Autodesk Inventor part; units mm, degrees
ref_plane "YZ Plane" through (0, 0, 0) normal (1, 0, 0) x (0, 1, 0)
ref_plane "XZ Plane" through (0, 0, 0) normal (0, 1, 0) x (-1, 0, 0)
ref_plane "XY Plane" through (0, 0, 0) normal (0, 0, 1) x (1, 0, 0)
sketch "Boceto1" plane through (0, 0, 0) normal (0, 0, 1) x (1, 0, 0)
  line L0 (0, 0) -> (50, 0)
  line L1 (50, 0) -> (50, 50)
  line L2 (50, 50) -> (0, 50)
  line L3 (0, 50) -> (0, 0)
  line L4 (50, 0) -> (0, 0)
  line L5 (0, 0) -> (0, 10)
  line L6 (0, 10) -> (50, 10)
  line L7 (50, 10) -> (50, 0)
  dimension "d0" = 50
  dimension "d1" = 50
  dimension "d2" = 10
extrude "Extrusión1" add sketch "Boceto1" along normal blind 10
sketch "Boceto2" plane through (0, 0, 10) normal (0, 0, 1) x (1, 0, 0)
  line L0 (0, 0) -> (50, 0)
  line L1 (0, 50) -> (0, 0)
  line L2 (50, 0) -> (0, 0)
  line L3 (0, 0) -> (0, 10)
  line L4 (0, 10) -> (50, 10)
  line L5 (50, 10) -> (50, 0)
  dimension "d5" = 10
extrude "Extrusión2" add sketch "Boceto2" along normal blind 30
sketch "Boceto3" plane through (0, 0, 10) normal (0, 0, 1) x (1, 0, 0)
  circle A0 centre (25, 25) radius 3.4
  line L0 (0, 50) -> (0, 10)
  line L1 (0, 0) -> (50, 0)
  dimension "d8" = 6.8
  dimension "d9" = 25
  dimension "d10" = 25
extrude "Extrusión3" cut sketch "Boceto3" against normal blind 10
sketch "Boceto4" plane through (0, 10, 10) normal (0, 1, 0) x (1, 0, 0)
  circle A0 centre (25, -20) radius 5.1
  line L0 (50, 10) -> (0, 10)
  line L1 (0, 0) -> (0, -30)
  dimension "d13" = 10.2
  dimension "d14" = 30
  dimension "d15" = 25
extrude "Extrusión4" cut sketch "Boceto4" against normal blind 10
sketch "Boceto5" plane through (0, 0, 0) normal (-1, 0, 0) x (0, 0, 1)
  line L0 (0, 50) -> (10, 50)
  line L1 (10, 10) -> (40, 10)
  line L2 (10, 50) -> (40, 10)
  line L3 (40, 10) -> (10, 10)
  line L4 (10, 10) -> (10, 50)
  line L5 (10, 50) -> (10, 10)
  point P0 (0, 0)
extrude "Extrusión5" add sketch "Boceto5" against normal blind 5
sketch "Boceto6" plane through (50, 0, 0) normal (1, 0, 0) x (0, 0, -1)
  line L0 (-10, 50) -> (-40, 10)
  line L1 (-10, 10) -> (-40, 10)
  line L2 (-10, 50) -> (-40, 10)
  line L3 (-40, 10) -> (-10, 10)
  line L4 (-10, 50) -> (-10, 10)
  line L5 (-10, 10) -> (-10, 50)
  point P0 (0, 0)
sketch "Boceto7" plane through (50, 0, 0) normal (1, 0, 0) x (0, 0, -1)
  point P0 (0, 0)
sketch "Boceto8" plane through (0, 0, 10) normal (0, 0, 1) x (1, 0, 0)
  point P0 (0, 0)
extrude "Extrusión6" add sketch "Boceto6" against normal blind 5
sketch "Boceto9" plane through (0, 0, 0) normal (0, 0, -1) x (-1, 0, 0)
  line L0 (-5, 5) -> (-45, 5)
  line L1 (-45, 5) -> (-45, 45)
  line L2 (-45, 45) -> (-5, 45)
  line L3 (-5, 45) -> (-5, 5)
  line L4 (-50, 0) -> (-50, 50)
  line L5 (-50, 50) -> (0, 50)
  line L6 (0, 50) -> (0, 0)
  line L7 (0, 0) -> (-50, 0)
  line L8 (-50, 0) -> (-50, 50)
  line L9 (-50, 50) -> (0, 50)
  line L10 (0, 50) -> (0, 0)
extrude "Extrusión7" add sketch "Boceto9" along normal blind 20
sketch "Boceto10" plane through (50, 0, 40) normal (1, 0, 0) x (0, 0, -1)
  line L0 (0, 0) -> (0, 10)
  circle A0 centre (50, 25) radius 3.375
  line L1 (60, 0) -> (0, 0)
  line L2 (60, 50) -> (60, 0)
  point P0 (40, 0)
  dimension "d28" = 40
  dimension "d29" = 6.75
sketch "Boceto11" plane through (0, 0, 40) normal (0, -1, 0) x (1, 0, 0)
  circle A0 centre (25, -50) radius 3.375
  line L0 (0, -60) -> (0, 0)
  line L1 (50, -60) -> (0, -60)
  point P0 (0, -40)
  dimension "d32" = 6.75
sketch "Boceto12" plane through (0, 0, 40) normal (-1, 0, 0) x (0, 0, 1)
  circle A0 centre (-50, 25) radius 3.375
  line L0 (-60, 0) -> (-60, 50)
  line L1 (-30, 50) -> (-60, 50)
  point P0 (-40, 0)
  dimension "d35" = 6.75
sketch "Boceto13" plane through (0, 50, 10) normal (0, 1, 0) x (1, 0, 0)
  circle A0 centre (25, 20) radius 3.375
  line L0 (0, 30) -> (50, 30)
  line L1 (50, 30) -> (50, 0)
  point P0 (0, 10)
  dimension "d38" = 6.75
  dimension "d39" = 10
  dimension "d40" = 25
extrude "Extrusión8" cut sketch "Boceto13" against normal blind 5
extrude "Extrusión9" cut sketch "Boceto10" against normal blind 5
extrude "Extrusión10" cut sketch "Boceto11" against normal blind 5
extrude "Extrusión11" cut sketch "Boceto12" against normal blind 5
properties part number "UnionLlantaOmega" material "Plástico ABS"
Input: part model. Units: mm. Frame: model coordinates. A direction names the side the tool comes from. Give positions to 0.01 mm unless a question says otherwise; leave off trailing zeros. Write each loop counter-clockwise with the first axis right and the second up, starting at its lowest first coordinate (ties: lowest second). Pieces come first, ordered by that corner, then holes.
Q1. Set-up query: faces 1 (the face through (5, 21, 18)), 2 (the face through (25, 50, -5)), 3 (the face through (29, 5, -10)). Return all of +Z, -Z, +X, -X, +Y, -Y with unobstructed straight access to the full face (end or side cutting, diameter ignored); none if empty.
Q2. Material intervals for probe 1 along Z at (x, y) = (25, 4.5) (3 decimals); probe 2 along X at (y, z) = (21, 26), sorted ascending.
Q3. First-contact query: P1, Ø1, axis at x = 13, y = 38, coming from the +Z side; P2, Ø2, axis at x = 32.5, y = 23, coming from the -Z side; P3, Ø15, axis at x = 25.5, z = 20, coming from the +Y side; P4, Ø16, axis at y = 22.5, z = -10, coming from the -X side. Flat tips, straight axial feed; report the tip coordinate or a pass-through.
Q4. Section A-A, the plane x = 25. Output: boundary loops of the cut face in (y, z) (3 decimals), plus the area to 4 significant figures.
Q5. Section D-D, the plane y = 7.5. Output: boundary loops of the cut face in (x, z), plus the area to 3 significant figures.
Q6. Pull-direction query (X, two-part tool) for faces 4 (the face through (45, 29, -10)), 5 (the face through (0, 20, 4)), 6 (the face through (2, 30, 25)), 7 (the face through (20.95, 5.07, 33.1)); classes: pulls with the +X half, pulls with the -X half, needs draft (parallel to the pull), parting line crosses it, or undercut.
Q7. Section B-B, the plane y = 25. Output: boundary loops of the cut face in (x, z) (3 decimals), plus the area to 3 significant figures.
Q8. Section C-C, the plane z = -16. Output: boundary loops of the cut face in (x, y), plus the area to 3 significant figures.
Filled in:
1. face 1: +Z, +Y
1. face 2: +Z, -Z, +X, -X, +Y
1. face 3: -Z
2. probe 1: z = -20 to -13.375, -6.625 to 24.9, 35.1 to 40
2. probe 2: x = 0 to 5, 45 to 50
3. P1: stops at z = 10
3. P2: stops at z = 0
3. P3: stops at y = 10
3. P4: stops at x = 0
4. outline: (0, -20) - (5, -20) - (5, -13.375) - (0, -13.375) - close; (0, -6.625) - (5, -6.625) - (5, 0) - (21.6, 0) - (21.6, 10) - (10, 10) - (10, 24.9) - (0, 24.9) - close; (0, 35.1) - (10, 35.1) - (10, 40) - (0, 40) - close; (28.4, 0) - (45, 0) - (45, -6.625) - (50, -6.625) - (50, 10) - (28.4, 10) - close; (45, -20) - (50, -20) - (50, -13.375) - (45, -13.375) - close
4. area: 762.5 mm2
5. outline: (0, -20) - (5, -20) - (5, 0) - (45, 0) - (45, -20) - (50, -20) - (50, 40) - (0, 40) - close; hole circle Ø10.2 at (25, 30)
5. area: 2,120 mm2
6. face 4: undercut
6. face 5: pulls with the -X half
6. face 6: needs draft
6. face 7: undercut
7. outline: (0, -20) - (5, -20) - (5, -13.375) - (0, -13.375) - close; (0, -6.625) - (5, -6.625) - (5, 0) - (21.6, 0) - (21.6, 10) - (5, 10) - (5, 28.75) - (0, 28.75) - close; (28.4, 0) - (45, 0) - (45, -6.625) - (50, -6.625) - (50, 28.75) - (45, 28.75) - (45, 10) - (28.4, 10) - close; (45, -20) - (50, -20) - (50, -13.375) - (45, -13.375) - close
7. area: 752 mm2
8. outline: (0, 0) - (50, 0) - (50, 50) - (0, 50) - close; hole (5, 5) - (45, 5) - (45, 45) - (5, 45) - close
8. area: 900 mm2
